```python
from build123d import *

# Parameters (mm, degrees)
F1_DEPTH       = 8
F2_DEPTH       = 4
F3_D           = 1.5
F4_DEPTH       = 12
F5_D           = 3
F5_CSINK_D     = 6
F5_CSINK_ANGLE = 90


with BuildPart() as f1:
    # F0 (on Top) → F1 (new body)
    with BuildSketch(Plane.XY):
        with BuildLine():
            Line((8.227241336, 4.75), (9.5262794416, 5.5))
            ThreePointArc((9.5262794416, 5.5), (0, 11), (-9.5262794416, 5.5))
            Line((-9.5262794416, 5.5), (-8.227241336, 4.75))
            ThreePointArc((-8.227241336, 4.75), (0, 9.5), (8.227241336, 4.75))
        make_face()
    extrude(amount=F1_DEPTH)



with BuildPart() as f1b:
    # F0 (on Top) → F1, piece 2 (new body)
    with BuildSketch(Plane.XY):
        with BuildLine():
            ThreePointArc((-9.5262794416, -5.5), (0, -11), (9.5262794416, -5.5))
            Line((9.5262794416, -5.5), (8.227241336, -4.75))
            ThreePointArc((8.227241336, -4.75), (0, -9.5), (-8.227241336, -4.75))
            Line((-8.227241336, -4.75), (-9.5262794416, -5.5))
        make_face()
    extrude(amount=F1_DEPTH)


with BuildPart() as f1_1:
    add(f1.part)

    add(f1b.part)  # F2 merges F1b
    # F0 (on Top) → F2 (join)
    with BuildSketch(Plane.XY):
        with BuildLine():
            ThreePointArc((9.5, 0), (9.1762953497, 2.4587809285), (8.227241336, 4.75))
            ThreePointArc((8.227241336, 4.75), (0, 9.5), (-8.227241336, 4.75))
            ThreePointArc((-8.227241336, 4.75), (-9.5, 0), (-8.227241336, -4.75))
            ThreePointArc((-8.227241336, -4.75), (0, -9.5), (8.227241336, -4.75))
            ThreePointArc((8.227241336, -4.75), (9.1762953497, -2.4587809285), (9.5, 0))
        make_face()
    extrude(amount=F2_DEPTH)

    # F3 (through all)
    with Locations(Plane(origin=(0, 0, 0), x_dir=(1, 0, 0), z_dir=(0, 0, -1))):
        with Locations((2, 0), (-2, 0)):
            Hole(F3_D / 2)

    # F0 (on Top) → F4 (join)
    with BuildSketch(Plane.XY):
        with BuildLine():
            Line((-8.227241336, 4.75), (-9.5262794416, 5.5))
            ThreePointArc((-9.5262794416, 5.5), (-11, 0), (-9.5262794416, -5.5))
            Line((-9.5262794416, -5.5), (-8.227241336, -4.75))
            ThreePointArc((-8.227241336, -4.75), (-9.5, 0), (-8.227241336, 4.75))
        make_face()
        with BuildLine():
            ThreePointArc((9.5262794416, -5.5), (10.6251840892, -2.8470094961), (11, 0))
            ThreePointArc((11, 0), (10.6251840892, 2.8470094961), (9.5262794416, 5.5))
            Line((9.5262794416, 5.5), (8.227241336, 4.75))
            ThreePointArc((8.227241336, 4.75), (9.1762953497, 2.4587809285), (9.5, 0))
            ThreePointArc((9.5, 0), (9.1762953497, -2.4587809285), (8.227241336, -4.75))
            Line((8.227241336, -4.75), (9.5262794416, -5.5))
        make_face()
    extrude(amount=F4_DEPTH)

    # F5 (through all)
    with Locations(Plane(origin=(0, 0, 0), x_dir=(1, 0, 0), z_dir=(0, 0, -1))):
        with Locations((0, 4), (0, -5.5)):
            CounterSinkHole(F5_D / 2, F5_CSINK_D / 2, counter_sink_angle=F5_CSINK_ANGLE)


solid = f1_1.part
```
Part model, mm, in its own coordinate system. A direction names the side the tool comes from. Round coordinates to 2 decimals unless told otherwise and drop trailing zeros. Write each loop counter-clockwise with the first axis right and the second up, starting at its lowest first coordinate (ties: lowest second). Pieces come first, ordered by that corner, then holes. Notation, with made-up numbers: (43, 44.25) -> (89, 44.25) arc R34 ccw to (89, 78.25) -> close; hole circle Ø8 at (58, 64). An arc over 180 degrees is marked (long way). Return JSON: item names as keys, results as strings. Group by question number.
Q1. Probe L1, parallel to X at y = 5.5, z = 2.1; L2, parallel to Y at x = 0.5, z = 3.75; L3, parallel to Z at x = -1.75, y = -1.5. List the from-to ranges inside material, lowest first. Write a range as [from, to].
Q2. Saw through at A-A on x = 0. Write the cut outline in (y, z), plus the area to 3 significant figures.
Q3. Which spindle directions (+Z, -Z, +X, -X, +Y, -Y) get a long thin tool onto all of the face, cutting with end or side? Do faces 1 (the flat face through (-10, 0, 12)), 2 (the flat face through (8.87, -5.12, 9.97)), 3 (the flat face through (-8.87, 5.12, 9.97)). Say none if no direction does.
Q4. Saw through at C-C on z = 3.25. Write the cut outline in (x, y), plus the area to 3 significant figures.
Q5. Saw through at B-B on z = 11. Write the cut outline in (x, y), plus the area to 3 significant figures.
Q6. Pin check, flat tips, straight feed: pin 1 (6 mm diameter, centred on x = -2.5, z = 9, fed in from -Y); pin 2 (5 mm diameter, centred on y = -7.5, z = 2.5, fed in from -X); pin 3 (4 mm diameter, centred on x = 2.5, y = 1, fed in from +Z); pin 4 (1 mm diameter, centred on y = 6, z = 1.5, fed in from -X). Stop position of each tip, or through.
Q7. Mould opens along X. For faces 4 (the flat face through (0, 0, 4)), 5 (the flat face through (8.886, 5.13, 9.972)), 6 (the flat face through (10, 0, 12)) say: pulls with the +X half, pulls with the -X half, needs draft (parallel to the pull), parting line crosses it, or undercut.
Q8. Saw through at D-D on z = 7. Write the cut outline in (x, y), plus the area to 3 significant figures.
Answer:
{
 "1": {"L1": "[-9.53, -1.5], [1.5, 9.53]", "L2": "[-10.99, -5.41], [-2.59, 4.09], [6.91, 10.99]", "L3": "[0, 4]"},
 "2": {"outline": "(-11, 0) -> (-7, 0) -> (-5.5, 1.5) -> (-5.5, 4) -> (-9.5, 4) -> (-9.5, 8) -> (-11, 8) -> close; (-2.5, 1.5) -> (-1, 0) -> (2.5, 0) -> (4, 1.5) -> (4, 4) -> (-2.5, 4) -> close; (7, 1.5) -> (8.5, 0) -> (11, 0) -> (11, 8) -> (9.5, 8) -> (9.5, 4) -> (7, 4) -> close", "area": "71.5 mm2"},
 "3": {"face 1": "+Z, +X, -X, +Y, -Y", "face 2": "+Z, -Y", "face 3": "+Z, +Y"},
 "4": {"outline": "circle Ø22 at (0, 0); hole circle Ø1.5 at (-2, 0); hole circle Ø3 at (0, -4); hole circle Ø3 at (0, 5.5); hole circle Ø1.5 at (2, 0)", "area": "362 mm2"},
 "5": {"outline": "(-9.53, -5.5) -> (-8.23, -4.75) arc R9.5 cw to (-8.23, 4.75) -> (-9.53, 5.5) arc R11 ccw to start; (8.23, -4.75) -> (9.53, -5.5) arc R11 ccw to (9.53, 5.5) -> (8.23, 4.75) arc R9.5 cw to start", "area": "32.2 mm2"},
 "6": {"pin 1": "y = -11", "pin 2": "x = -9.8", "pin 3": "z = 4", "pin 4": "x = -9.53"},
 "7": {"face 4": "undercut", "face 5": "undercut", "face 6": "needs draft"},
 "8": {"outline": "circle Ø22 at (0, 0); hole circle Ø19 at (0, 0)", "area": "96.6 mm2"}
}
